Autodesk Inventor part; units mm, degrees
ref_plane "YZ Plane" through (0, 0, 0) normal (1, 0, 0) x (0, 1, 0)
ref_plane "XZ Plane" through (0, 0, 0) normal (0, 1, 0) x (-1, 0, 0)
ref_plane "XY Plane" through (0, 0, 0) normal (0, 0, 1) x (1, 0, 0)
sketch "Sketch1" plane through (0, 0, 0) normal (0, 0, 1) x (1, 0, 0)
  line L0 (-85.48, 55.38) -> (85.48, 55.38)
  line L1 (96.48, 44.38) -> (96.48, -44.38)
  line L2 (85.48, -55.38) -> (-85.48, -55.38)
  line L3 (-96.48, -44.38) -> (-96.48, 44.38)
  arc A0 (-85.48, 55.38) -> (-96.48, 44.38) centre (-85.48, 44.38) ccw
  arc A1 (96.48, 44.38) -> (85.48, 55.38) centre (85.48, 44.38) ccw
  arc A2 (85.48, -55.38) -> (96.48, -44.38) centre (85.48, -44.38) ccw
  arc A3 (-96.48, -44.38) -> (-85.48, -55.38) centre (-85.48, -44.38) ccw
  point P0 (0, 0)
  point P1 (-96.48, 55.38)
  point P2 (96.48, 55.38)
  point P3 (-96.48, -55.38)
  dimension "d0" = 192.96
  dimension "d1" = 110.76
  dimension "d2" = 96.48
  dimension "d3" = 55.38
  dimension "d6" = 11
extrude "Extrusion2" add sketch "Sketch1" along normal blind 1
sketch "Sketch3" plane through (0, 0, 0) normal (0, 0, -1) x (-1, 0, 0)
  line L0 (-83.1, 48.75) -> (83.1, 48.75)
  line L1 (83.1, 48.75) -> (83.1, -51.85)
  line L2 (83.1, -51.85) -> (-83.1, -51.85)
  line L3 (-83.1, -51.85) -> (-83.1, 48.75)
  line L4 (85.48, 55.38) -> (-85.48, 55.38)
  point P0 (0, 0)
  dimension "d9" = 166.2
  dimension "d10" = 100.6
  dimension "d12" = 83.1
  dimension "d13" = 6.63
extrude "Extrusion3" add sketch "Sketch3" along normal blind 4.96
sketch "Sketch4" plane through (0, 0, -4.96) normal (0, 0, -1) x (-1, 0, 0)
  line L0 (-70.6, 37.8) -> (-55.6, 37.8)
  line L1 (-55.6, 37.8) -> (-55.6, 29.8)
  line L2 (-55.6, 29.8) -> (-70.6, 29.8)
  line L3 (-70.6, 29.8) -> (-70.6, 37.8)
  circle A0 centre (-63.1, 33.8) radius 1.5
  line L4 (-83.1, 48.75) -> (-83.1, -51.85)
  line L5 (55.6, 37.8) -> (70.6, 37.8)
  circle A1 centre (63.1, 33.8) radius 1.5
  line L6 (55.6, 29.8) -> (55.6, 37.8)
  line L7 (70.6, 29.8) -> (55.6, 29.8)
  line L8 (70.6, 37.8) -> (70.6, 29.8)
  line L9 (-70.6, -27.85) -> (-55.6, -27.85)
  circle A2 centre (-63.1, -31.85) radius 1.5
  line L10 (-70.6, -35.85) -> (-70.6, -27.85)
  line L11 (-55.6, -35.85) -> (-70.6, -35.85)
  line L12 (-55.6, -27.85) -> (-55.6, -35.85)
  line L13 (55.6, -27.85) -> (70.6, -27.85)
  circle A3 centre (63.1, -31.85) radius 1.5
  line L14 (55.6, -35.85) -> (55.6, -27.85)
  line L15 (70.6, -35.85) -> (55.6, -35.85)
  line L16 (70.6, -27.85) -> (70.6, -35.85)
  line L17 (83.1, 48.75) -> (-83.1, 48.75)
  line L18 (-38.65, 20.45) -> (-38.65, 35.45)
  circle A4 centre (-34.65, 27.95) radius 1.25
  line L19 (-30.65, 20.45) -> (-38.65, 20.45)
  line L20 (-30.65, 35.45) -> (-30.65, 20.45)
  line L21 (-38.65, 35.45) -> (-30.65, 35.45)
  line L22 (83.1, -51.85) -> (83.1, 48.75)
  line L23 (85.48, 55.38) -> (-85.48, 55.38)
  line L24 (19.35, 20.45) -> (19.35, 35.45)
  line L25 (19.35, 35.45) -> (27.35, 35.45)
  line L26 (27.35, 35.45) -> (27.35, 20.45)
  line L27 (27.35, 20.45) -> (19.35, 20.45)
  circle A5 centre (23.35, 27.95) radius 1.25
  line L28 (-38.65, -28.55) -> (-38.65, -13.55)
  line L29 (-38.65, -13.55) -> (-30.65, -13.55)
  line L30 (-30.65, -13.55) -> (-30.65, -28.55)
  line L31 (-30.65, -28.55) -> (-38.65, -28.55)
  circle A6 centre (-34.65, -21.05) radius 1.25
  line L32 (19.35, -28.55) -> (19.35, -13.55)
  line L33 (19.35, -13.55) -> (27.35, -13.55)
  line L34 (27.35, -13.55) -> (27.35, -28.55)
  line L35 (27.35, -28.55) -> (19.35, -28.55)
  circle A7 centre (23.35, -21.05) radius 1.25
  point P0 (0, 0)
  point P1 (-55.6, 33.8)
  point P2 (-63.1, 37.8)
  point P3 (63.1, 37.8)
  point P4 (70.6, 33.8)
  point P5 (-63.1, -27.85)
  point P6 (-55.6, -31.85)
  point P7 (63.1, -27.85)
  point P8 (70.6, -31.85)
  point P9 (64.6875, 33.5375)
  point P10 (72.1875, 29.5375)
  point P11 (-38.65, 27.95)
  point P12 (-34.65, 35.45)
  point P13 (122.6875, 33.5375)
  point P14 (19.35, 27.95)
  point P15 (130.1875, 29.5375)
  point P16 (23.35, 35.45)
  point P17 (64.6875, -15.4625)
  point P18 (-38.65, -21.05)
  point P19 (72.1875, -19.4625)
  point P20 (-34.65, -13.55)
  point P21 (122.6875, -15.4625)
  point P22 (19.35, -21.05)
  point P23 (130.1875, -19.4625)
  point P24 (23.35, -13.55)
  dimension "d16" = 15
  dimension "d17" = 8
  dimension "d18" = 3
  dimension "d19" = 20
  dimension "d22" = 126.2
  dimension "d25" = 65.65
  dimension "d29" = 2.5
  dimension "d30" = 20.8
  dimension "d32" = 48.45
  dimension "d33" = 21.58
  dimension "d44" = 58
  dimension "d47" = 49
extrude "Extrusion4" add sketch "Sketch4" along normal blind 2.5
chamfer "Chamfer1" distance 2.5 angle 45 16 edges at (70.6, 33.8, -7.46) (55.6, 33.8, -7.46) (34.65, 35.45, -7.46) (34.65, 20.45, -7.46) (-23.35, 35.45, -7.46) (-23.35, 20.45, -7.46) (-55.6, 33.8, -7.46) (-70.6, 33.8, -7.46) (70.6, -31.85, -7.46) (55.6, -31.85, -7.46) (34.65, -13.55, -7.46) (34.65, -28.55, -7.46) (-23.35, -13.55, -7.46) (-23.35, -28.55, -7.46) (-55.6, -31.85, -7.46) (-70.6, -31.85, -7.46)
sketch "Sketch5" plane through (0, 0, 1) normal (0, 0, 1) x (1, 0, 0)
  line L0 (-77.5, 43.5) -> (77.5, 43.5)
  line L1 (77.5, 43.5) -> (77.5, -43.5)
  line L2 (77.5, -43.5) -> (-77.5, -43.5)
  line L3 (-77.5, -43.5) -> (-77.5, 43.5)
  point P0 (0, 0)
  dimension "d55" = 155
  dimension "d56" = 87
  dimension "d57" = 43.5
  dimension "d58" = 77.5
extrude "Extrusion5" add sketch "Sketch5" along normal blind 0.01
properties part number "Touchscreen"
Source: CAD feature listing. Evaluate the final solid. Frame: model axes, mm. A direction names the side the tool comes from. Round coordinates to 2 decimals unless told otherwise and drop trailing zeros. Loops run counter-clockwise (first coordinate to the right, second up) from the corner with the lowest first, then second, coordinate; pieces in that order, holes last.
(1) Section query C-C (z = -1.75). Output: boundary loops of the cut face in (x, y), and give its area (3 significant figures).
From the geometry:
outline: (-83.1, -51.85) - (83.1, -51.85) - (83.1, 48.75) - (-83.1, 48.75) - close
area: 16,700 mm2
(2) Pull-direction query (X, two-part tool) for faces 4 (the flat face through (1, -1, -4.96)), 5 (the flat face through (63, -30, -7.46)), 6 (the cylindrical face through (93.172, 52.243, 0.493)); classes: +X half, -X half, draft (parallel to the pull), parting line (faces both ways), or undercut.
From the geometry:
face 4: undercut
face 5: draft
face 6: +X half
(3) Access query for faces 1 (the flat face through (-83.1, -1, -2)), 2 (the flat face through (0, 49, 0)), 3 (the flat face through (-1, -51.85, -2)). Directions: +Z, -Z, +X, -X, +Y, -Y. A direction counts if a zero-diameter tool reaches every point of the face in a straight line with its end or side. Return the directions, or none.
From the geometry:
face 1: -Z, -X, +Y, -Y
face 2: -Z
face 3: -Z, +X, -X, -Y
(4) Material intervals for probe 1 along Y at (x, z) = (34.65, -6.35); probe 2 along X at (y, z) = (33.5, -5); probe 3 along Y at (x, z) = (-63.1, -5.9), sorted ascending.
From the geometry:
probe 1: y = -27.16 to -22.3, -19.8 to -14.94, 21.84 to 26.7, 29.2 to 34.06
probe 2: x = -70.56 to -64.57, -61.63 to -55.64, -27.35 to -19.35, 30.65 to 38.65, 55.64 to 61.63, 64.57 to 70.56
probe 3: y = -35.85 to -33.35, -30.35 to -27.85, 29.8 to 32.3, 35.3 to 37.8
(5) Contact query for flat-ended pins moving along their axis: pin 1 Ø5 at (y, z) = (-1, -4.5) entering from +X; pin 2 Ø2 at (y, z) = (-18, -6.5) entering from +X; pin 3 Ø4 at (y, z) = (-35.5, -2.5) entering from -X; pin 4 Ø5 at (x, z) = (0.5, -0.5) entering from +Y. Output: stop coordinate, or through.
From the geometry:
pin 1: stops at x = 83.1
pin 2: stops at x = 38.65
pin 3: stops at x = -83.1
pin 4: stops at y = 55.38
